from build123d import *

# Parameters (mm, degrees)
BOSS_EXTRUDE1_DEPTH             = 5
BOSS_EXTRUDE2_DEPTH             = 20
TAP_DRILL_FOR_M3X0_5_TAP1_D     = 2.5
TAP_DRILL_FOR_M3X0_5_TAP1_DEPTH = 6
TAP_DRILL_FOR_M3X0_5_TAP1_TIP   = 0.751075774


with BuildPart() as part:
    # Sketch1 → Boss-Extrude1 (new body)
    with BuildSketch(Plane(origin=(0, 0, 0), x_dir=(1, 0, 0), z_dir=(0, 1, 0))):
        with BuildLine():
            Line((21, 27.921142965), (21, 72.078857035))
            ThreePointArc((21, 72.078857035), (20.927086518, 72.453704455), (20.718978822, 72.773889015))
            Line((20.718978822, 72.773889015), (6.281021178, 87.709296434))
            ThreePointArc((6.281021178, 87.709296434), (6.072913482, 88.029480993), (6, 88.404328413))
            Line((6, 88.404328413), (6, 93))
            ThreePointArc((6, 93), (6.292893219, 93.707106781), (7, 94))
            Line((7, 94), (11.575831706, 94))
            ThreePointArc((11.575831706, 94), (11.966323717, 93.920606316), (12.294810529, 93.69503198))
            Line((12.294810529, 93.69503198), (26.579929079, 78.91772962))
            ThreePointArc((26.579929079, 78.91772962), (50, 68.488702878), (73.420070921, 78.91772962))
            Line((73.420070921, 78.91772962), (87.705189471, 93.69503198))
            ThreePointArc((87.705189471, 93.69503198), (88.033676283, 93.920606316), (88.424168294, 94))
            Line((88.424168294, 94), (93, 94))
            ThreePointArc((93, 94), (93.707106781, 93.707106781), (94, 93))
            Line((94, 93), (94, 88.404328413))
            ThreePointArc((94, 88.404328413), (93.927086518, 88.029480993), (93.718978822, 87.709296434))
            Line((93.718978822, 87.709296434), (79.281021178, 72.773889015))
            ThreePointArc((79.281021178, 72.773889015), (79.072913482, 72.453704455), (79, 72.078857035))
            Line((79, 72.078857035), (79, 27.921142965))
            ThreePointArc((79, 27.921142965), (79.072913482, 27.546295545), (79.281021178, 27.226110985))
            Line((79.281021178, 27.226110985), (93.718978822, 12.290703566))
            ThreePointArc((93.718978822, 12.290703566), (93.927086518, 11.970519007), (94, 11.595671587))
            Line((94, 11.595671587), (94, 7))
            ThreePointArc((94, 7), (93.707106781, 6.292893219), (93, 6))
            Line((93, 6), (88.424168294, 6))
            ThreePointArc((88.424168294, 6), (88.033676283, 6.079393684), (87.705189471, 6.30496802))
            Line((87.705189471, 6.30496802), (73.420070921, 21.08227038))
            ThreePointArc((73.420070921, 21.08227038), (72.67313409, 21.386847499), (71.944389028, 21.040997121))
            ThreePointArc((71.944389028, 21.040997121), (50, 11), (28.055610972, 21.040997121))
            ThreePointArc((28.055610972, 21.040997121), (27.32686591, 21.386847499), (26.579929079, 21.08227038))
            Line((26.579929079, 21.08227038), (12.294810529, 6.30496802))
            ThreePointArc((12.294810529, 6.30496802), (11.966323717, 6.079393684), (11.575831706, 6))
            Line((11.575831706, 6), (7, 6))
            ThreePointArc((7, 6), (6.292893219, 6.292893219), (6, 7))
            Line((6, 7), (6, 11.595671587))
            ThreePointArc((6, 11.595671587), (6.072913482, 11.970519007), (6.281021178, 12.290703566))
            Line((6.281021178, 12.290703566), (20.718978822, 27.226110985))
            ThreePointArc((20.718978822, 27.226110985), (20.927086518, 27.546295545), (21, 27.921142965))
        make_face()
        with BuildLine():
            Line((27.5, 40), (27.5, 60))
            Line((27.5, 60), (72.5, 60))
            Line((72.5, 60), (72.5, 40))
            ThreePointArc((72.5, 40), (50, 17.5), (27.5, 40))
        make_face(mode=Mode.SUBTRACT)
    extrude(amount=BOSS_EXTRUDE1_DEPTH)

    # Sketch2 → Boss-Extrude2 (add)
    with BuildSketch(Plane(origin=(0, 5, 0), x_dir=(1, 0, 0), z_dir=(0, 1, 0))):
        with BuildLine():
            Line((11.575831706, 94), (7, 94))
            ThreePointArc((7, 94), (6.292893219, 93.707106781), (6, 93))
            Line((6, 93), (6, 88.404328413))
            ThreePointArc((6, 88.404328413), (6.072913482, 88.029480993), (6.281021178, 87.709296434))
            Line((6.281021178, 87.709296434), (6.671882728, 87.30496802))
            ThreePointArc((6.671882728, 87.30496802), (7.00036954, 87.079393684), (7.390861551, 87))
            Line((7.390861551, 87), (12, 87))
            ThreePointArc((12, 87), (12.707106781, 87.292893219), (13, 88))
            Line((13, 88), (13, 92.561217283))
            ThreePointArc((13, 92.561217283), (12.927086518, 92.936064704), (12.718978822, 93.256249263))
            Line((12.718978822, 93.256249263), (12.294810529, 93.69503198))
            ThreePointArc((12.294810529, 93.69503198), (11.966323717, 93.920606316), (11.575831706, 94))
        make_face()
        with BuildLine():
            Line((87, 88), (87, 92.561217283))
            ThreePointArc((87, 92.561217283), (87.072913482, 92.936064704), (87.281021178, 93.256249263))
            Line((87.281021178, 93.256249263), (87.705189471, 93.69503198))
            ThreePointArc((87.705189471, 93.69503198), (88.033676283, 93.920606316), (88.424168294, 94))
            Line((88.424168294, 94), (93, 94))
            ThreePointArc((93, 94), (93.707106781, 93.707106781), (94, 93))
            Line((94, 93), (94, 88.404328413))
            ThreePointArc((94, 88.404328413), (93.927086518, 88.029480993), (93.718978822, 87.709296434))
            Line((93.718978822, 87.709296434), (93.328117272, 87.30496802))
            ThreePointArc((93.328117272, 87.30496802), (92.99963046, 87.079393684), (92.609138449, 87))
            Line((92.609138449, 87), (88, 87))
            ThreePointArc((88, 87), (87.292893219, 87.292893219), (87, 88))
        make_face()
        with BuildLine():
            Line((88.424168294, 6), (93, 6))
            ThreePointArc((93, 6), (93.707106781, 6.292893219), (94, 7))
            Line((94, 7), (94, 11.595671587))
            ThreePointArc((94, 11.595671587), (93.927086518, 11.970519007), (93.718978822, 12.290703566))
            Line((93.718978822, 12.290703566), (93.328117272, 12.69503198))
            ThreePointArc((93.328117272, 12.69503198), (92.99963046, 12.920606316), (92.609138449, 13))
            Line((92.609138449, 13), (88, 13))
            ThreePointArc((88, 13), (87.292893219, 12.707106781), (87, 12))
            Line((87, 12), (87, 7.438782717))
            ThreePointArc((87, 7.438782717), (87.072913482, 7.063935296), (87.281021178, 6.743750737))
            Line((87.281021178, 6.743750737), (87.705189471, 6.30496802))
            ThreePointArc((87.705189471, 6.30496802), (88.033676283, 6.079393684), (88.424168294, 6))
        make_face()
        with BuildLine():
            Line((13, 12), (13, 7.438782717))
            ThreePointArc((13, 7.438782717), (12.927086518, 7.063935296), (12.718978822, 6.743750737))
            Line((12.718978822, 6.743750737), (12.294810529, 6.30496802))
            ThreePointArc((12.294810529, 6.30496802), (11.966323717, 6.079393684), (11.575831706, 6))
            Line((11.575831706, 6), (7, 6))
            ThreePointArc((7, 6), (6.292893219, 6.292893219), (6, 7))
            Line((6, 7), (6, 11.595671587))
            ThreePointArc((6, 11.595671587), (6.072913482, 11.970519007), (6.281021178, 12.290703566))
            Line((6.281021178, 12.290703566), (6.671882728, 12.69503198))
            ThreePointArc((6.671882728, 12.69503198), (7.00036954, 12.920606316), (7.390861551, 13))
            Line((7.390861551, 13), (12, 13))
            ThreePointArc((12, 13), (12.707106781, 12.707106781), (13, 12))
        make_face()
    extrude(amount=BOSS_EXTRUDE2_DEPTH)

    # Tap Drill for M3x0.5 Tap1
    with Locations(Plane(origin=(24.25, 5, -50), x_dir=(0, 0, 1), z_dir=(0, 1, 0))):
        with Locations((0, 0), (0, 51.5)):
            Hole(TAP_DRILL_FOR_M3X0_5_TAP1_D / 2, depth=TAP_DRILL_FOR_M3X0_5_TAP1_DEPTH)
            with Locations((0, 0, -(TAP_DRILL_FOR_M3X0_5_TAP1_DEPTH + TAP_DRILL_FOR_M3X0_5_TAP1_TIP / 2))):  # 118° drill point
                Cone(0, TAP_DRILL_FOR_M3X0_5_TAP1_D / 2, TAP_DRILL_FOR_M3X0_5_TAP1_TIP, mode=Mode.SUBTRACT)


solid = part.part
For this review, take the finished solid that the model builds, in its own axes (mm). A direction names the side the tool comes from. Round coordinates to 2 decimals unless told otherwise and drop trailing zeros. Write each loop counter-clockwise with the first axis right and the second up, starting at its lowest first coordinate (ties: lowest second). Pieces come first, ordered by that corner, then holes. Notation, with made-up numbers: (75.5, -11) -> (111.5, -11) arc R25 ccw to (111.5, 25) -> close; hole circle Ø8 at (88, -24). An arc over 180 degrees is marked (long way). Use CSV: the item, a comma, the result in double quotes.
(1) To check wall thickness, follow L1, parallel to X at y = 2.75, z = -50; L2, parallel to Z at x = 11, y = 22.5; L3, parallel to X at y = 1.75, z = -78.5. State the ranges of each line that lie inside material, in increasing order. Write a range as [from, to].
Computed values:
L1,"[21, 23], [25.5, 27.5], [72.5, 74.5], [77, 79]"
L2,"[-94, -87], [-13, -6]"
L3,"[15.18, 26.96], [73.04, 84.82]"
(2) Consider section C-C, the plane z = -38.5. Give the boundary of the cut face in (x, y), plus the area to 3 significant figures.
Computed values:
outline,"(21, 0) -> (27.55, 0) -> (27.55, 5) -> (21, 5) -> close; (72.45, 0) -> (79, 0) -> (79, 5) -> (72.45, 5) -> close"
area,"65.5 mm²"
(3) For faces 1 (the face through (21, 2, -50)), 2 (the face through (13, 15, -10)), 3 (the face through (90, 15, -13)), 4 (the face through (50, 2, -60)), 5 (the face through (79, 2, -50)), list the 3-axis set-ups (+Z, -Z, +X, -X, +Y, -Y) from which the entire face can be reached by the end or side of a thin tool; tool diameter is ignored.
Computed values:
face 1,"-X, +Y, -Y"
face 2,"+Z, -Z, +Y"
face 3,"+X, -X, +Y"
face 4,"+Y, -Y"
face 5,"+X, +Y, -Y"
(4) Draft analysis for pull direction Z (two halves, no side actions). For faces 6 (the face through (94, 12, -91)), 7 (the face through (91, 12, -94)), 8 (the face through (10, 15, -87)), state which applies: +Z half, -Z half, draft (parallel to the pull), parting line (faces both ways), or undercut.
Computed values:
face 6,"draft"
face 7,"-Z half"
face 8,"undercut"
(5) Consider section A-A, the plane z = -50. Give the boundary of the cut face in (x, y).
Computed values:
outline,"(21, 0) -> (23, 0) -> (23, 5) -> (21, 5) -> close; (25.5, 0) -> (27.5, 0) -> (27.5, 5) -> (25.5, 5) -> close; (72.5, 0) -> (74.5, 0) -> (74.5, 5) -> (72.5, 5) -> close; (77, 0) -> (79, 0) -> (79, 5) -> (77, 5) -> close"
(6) Consider section B-B, the plane x = 50. Give the boundary of the cut face in (y, z), plus the area to 3 significant figures.
Computed values:
outline,"(0, -68.49) -> (5, -68.49) -> (5, -60) -> (0, -60) -> close; (0, -17.5) -> (5, -17.5) -> (5, -11) -> (0, -11) -> close"
area,"74.9 mm²"
(7) Clearance check with flat-ended pins moving along their axes: P1, Ø1.5, axis at x = 80.5, z = -22.5, coming from the +Y side; P2, Ø10, axis at x = 20.5, y = 6.5, coming from the -Z side; P3, Ø1.5, axis at y = 3.5, z = -57.5, coming from the -X side; P4, Ø1, axis at y = 6.5, z = -67.5, coming from the -X side. State where each tip first meets the part, or that it passes through.
Computed values:
P1,"y = 5"
P2,"z = -90.14"
P3,"x = 21"
P4,"through"
(8) Consider section D-D, the plane y = 10.25. Give the number of separate pieces and of enclosed holes in the cut face, plus the area to 3 significant figures.
Computed values:
separate pieces,"4"
enclosed holes,"0"
area,"190 mm²"
